Can you work these out from the model? Positions are in its coordinate system, mm. Round coordinates to 2 decimals unless told otherwise and drop trailing zeros. Write each loop counter-clockwise with the first axis right and the second up, starting at its lowest first coordinate (ties: lowest second). Pieces come first, ordered by that corner, then holes.
Q1. Please list where these lines run through material, in increasing order: line 1 along Y through (x, z) = (0, 3.75); line 2 along X through (y, z) = (-9, 3.75); line 3 along X through (y, z) = (-12, 5.75).
Q2. If we section it at A-A (x = 0): Please give me the cut outline in (y, z).
Q3. I'm going to push flat-ended pins straight in: pin 1 Ø2 at (x, y) = (-61.5, 14.5) entering from -Z; pin 2 Ø2 at (y, z) = (4.5, 3) entering from +X. Where does each tip first touch, or does it pass through?
Q4. If we section it at D-D (x = 83.5): Please give me the cut outline in (y, z).
Q5. If we section it at B-B (y = 6): Please give me the cut outline in (x, z), plus the area to 3 significant figures.
Q6. We'd pull the mould along X, two halves only. Please class faces 1 (the flat face through (1, -19.05, 3)), 2 (the cylindrical face through (114.295, 0.419, 3.131)), 3 (the cylindrical face through (-0.44, 10.73, 3.13)): +X half, -X half, draft (parallel to the pull), parting line (faces both ways), or undercut.
Q7. If we section it at C-C (z = 4.5): Give the number of separate pieces and of enclosed holes in the cut face, plus the area to 3 significant figures.
from build123d import *

# Parameters (mm, degrees)
SKETCH1_R           = 14.2875
SKETCH1_R_2         = 2.0193
BOSS_EXTRUDE1_DEPTH = 6.35


with BuildPart() as part:
    # Sketch1 → Boss-Extrude1 (new body)
    with BuildSketch(Plane.XY):
        with BuildLine():
            Line((-95.25, 19.05), (95.25, 19.05))
            ThreePointArc((95.25, 19.05), (114.3, 0), (95.25, -19.05))
            Line((95.25, -19.05), (-95.25, -19.05))
            ThreePointArc((-95.25, -19.05), (-114.3, 0), (-95.25, 19.05))
        make_face()
        with Locations((-95.25, 0)):
            Circle(SKETCH1_R, mode=Mode.SUBTRACT)
        with Locations((95.25, 0)):
            Circle(SKETCH1_R, mode=Mode.SUBTRACT)
        with Locations((0, 12.7)):
            Circle(SKETCH1_R_2, mode=Mode.SUBTRACT)
        Circle(SKETCH1_R_2, mode=Mode.SUBTRACT)
        with Locations((0, -12.7)):
            Circle(SKETCH1_R_2, mode=Mode.SUBTRACT)
    extrude(amount=BOSS_EXTRUDE1_DEPTH)


solid = part.part
A:
1. line 1: y = -19.05 to -14.72, -10.68 to -2.02, 2.02 to 10.68, 14.72 to 19.05
1. line 2: x = -112.04 to -106.35, -84.15 to 84.15, 106.35 to 112.04
1. line 3: x = -110.05 to -103, -87.5 to -1.89, 1.89 to 87.5, 103 to 110.05
2. outline: (-19.05, 0) - (-14.72, 0) - (-14.72, 6.35) - (-19.05, 6.35) - close; (-10.68, 0) - (-2.02, 0) - (-2.02, 6.35) - (-10.68, 6.35) - close; (2.02, 0) - (10.68, 0) - (10.68, 6.35) - (2.02, 6.35) - close; (14.72, 0) - (19.05, 0) - (19.05, 6.35) - (14.72, 6.35) - close
3. pin 1: stops at z = 0
3. pin 2: stops at x = 113.98
4. outline: (-19.05, 0) - (-8.13, 0) - (-8.13, 6.35) - (-19.05, 6.35) - close; (8.13, 0) - (19.05, 0) - (19.05, 6.35) - (8.13, 6.35) - close
5. outline: (-113.33, 0) - (-108.22, 0) - (-108.22, 6.35) - (-113.33, 6.35) - close; (-82.28, 0) - (82.28, 0) - (82.28, 6.35) - (-82.28, 6.35) - close; (108.22, 0) - (113.33, 0) - (113.33, 6.35) - (108.22, 6.35) - close
5. area: 1,110 mm2
6. face 1: draft
6. face 2: +X half
6. face 3: undercut
7. separate pieces: 1
7. enclosed holes: 5
7. area: 7,080 mm2
